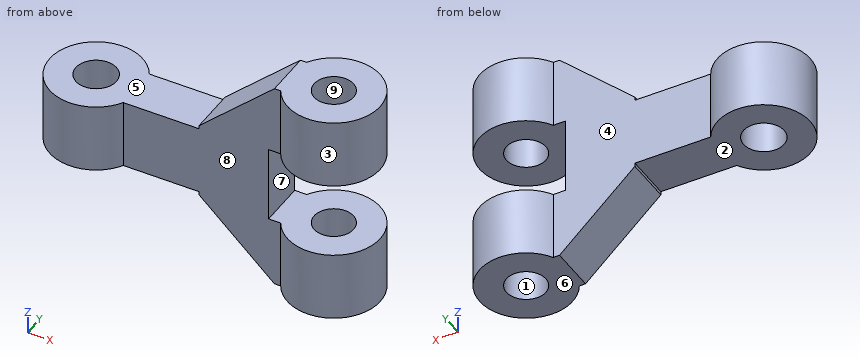
from build123d import *

# Parameters (mm, degrees)
SKETCH_1_R           = 4
SKETCH_1_R_2         = 1.7
EXTRUDE_1_DEPTH      = 6
EXTRUDE_2_DEPTH      = 2
EXTRUDE_2_DEPTH_BACK = 2
SKETCH_3_R           = 1.75
EXTRUDE_3_DEPTH      = 3
EXTRUDE_3_DEPTH_BACK = 3


with BuildPart() as part:
    # Sketch 1 → Extrude 1 (new body)
    with BuildSketch(Plane.XY):
        Circle(SKETCH_1_R)
        Circle(SKETCH_1_R_2, mode=Mode.SUBTRACT)
    extrude_1 = extrude(amount=EXTRUDE_1_DEPTH)

    # Sketch 2 → Extrude 2 (add, two sides)
    with BuildSketch(Plane(origin=(0, 0, 0), x_dir=(1, 0, 0), z_dir=(0, 1, 0))) as extrude_2_sk:
        Polygon((-4, 0), (-10.5, -6), (-10.5, -12.6), (-4, -18.6), (-3, -18.6), (-3, -12.6), (-4, -12.6), (-4.5, -12.6), (-4.5, -6), (-4, -6), (-3, -6), (-3, 0), align=None)
    extrude(amount=EXTRUDE_2_DEPTH)
    extrude(extrude_2_sk.sketch, amount=-EXTRUDE_2_DEPTH_BACK)

    # Mirror 1: Extrude 1 across plane
    add(extrude_1.mirror(Plane(origin=(0, 0, 9.3), x_dir=(1, 0, 0), z_dir=(0, 0, -1))))

    # Sketch 3 → Extrude 3 (add, two sides)
    with BuildSketch(Plane(origin=(0, 0, 9.3), x_dir=(-1, 0, 0), z_dir=(0, 0, -1))) as extrude_3_sk:
        with BuildLine():
            Line((10.5, 2), (17.035898385, 2))
            ThreePointArc((17.035898385, 2), (24.5, 0), (17.035898385, -2))
            Line((17.035898385, -2), (10.5, -2))
            Line((10.5, -2), (10.5, 2))
        make_face()
        with Locations((20.5, 0)):
            Circle(SKETCH_3_R, mode=Mode.SUBTRACT)
    extrude(amount=EXTRUDE_3_DEPTH)
    extrude(extrude_3_sk.sketch, amount=-EXTRUDE_3_DEPTH_BACK)


solid = part.part
Input: part model. Units: mm. Frame: model coordinates. Face numbers are marked on the shaded views. A direction names the side the tool comes from. Round coordinates to 2 decimals unless told otherwise and drop trailing zeros. Order: outer loops, then holes, each group sorted by start corner. A loop starts at its lowest first (then second) coordinate and runs counter-clockwise, first axis right, second up. Notation, with made-up numbers: (32, 16) - (70, 16) arc R26 cw to (70, 55) - close; hole circle Ø4 at (87.5, 74). An arc over 180 degrees is marked (long way). Answer as a JSON object with one key per item and string values. Group by question number.
(1) Material intervals for probe 1 along Z at (x, y) = (-3.25, 0.25); probe 2 along Y at (x, z) = (0, 15.1); probe 3 along X at (y, z) = (0.5, 11), sorted ascending. Write a range as from..to.
(2) Cut plane C-C (x = 0). Return loops of the section in (y, z), then the cut area to 3 significant figures.
(3) Reachability of the marked faces 5, 6, 7, 8 and 9 from +Z, -Z, +X, -X, +Y, -Y: full face, straight path, thin tool, end or side. Return the list, or none.
(4) Cut plane D-D (z = 11). Return loops of the section in (x, y).
(5) Cut plane B-B (y = 0). Return loops of the section in (x, z).
(6) Cut plane A-A (x = -20.5). Return loops of the section in (y, z), then the cut area to 3 significant figures.
(7) Draft query along Y for the marked faces 1, 2, 3 and 4. Return one class per face: released by +Y, released by -Y, zero draft, split by the parting line, or undercut.
(8) Pin query (flat end, axial travel): P1, Ø2, axis at y = -0.5, z = 10.5, coming from the +X side; P2, Ø4, axis at x = -13, z = 9.5, coming from the +Y side; P3, Ø4, axis at x = -10.5, z = 15, coming from the -Y side. Return the tip coordinate at first contact, or that it passes through.
Here are the results:
{
 "1": {"probe 1": "z = 0..6, 12.6..18.6", "probe 2": "y = -4..-1.7, 1.7..4", "probe 3": "x = -24.47..-22.18, -18.82..-4.5"},
 "2": {"outline": "(-4, 0) - (-1.7, 0) - (-1.7, 6) - (-4, 6) - close; (-4, 12.6) - (-1.7, 12.6) - (-1.7, 18.6) - (-4, 18.6) - close; (1.7, 0) - (4, 0) - (4, 6) - (1.7, 6) - close; (1.7, 12.6) - (4, 12.6) - (4, 18.6) - (1.7, 18.6) - close", "area": "55.2 mm^2"},
 "3": {"face 5": "+Z, -X, +Y, -Y", "face 6": "-Z, +X, -X, +Y, -Y", "face 7": "+X, +Y, -Y", "face 8": "+Z, -Z, -Y", "face 9": "+Z, -Z"},
 "4": {"outline": "(-17.04, -2) - (-4.5, -2) - (-4.5, 2) - (-17.04, 2) arc R4 ccw (long way) to start; hole circle Ø3.5 at (-20.5, 0)"},
 "5": {"outline": "(-24.5, 6.3) - (-22.25, 6.3) - (-22.25, 12.3) - (-24.5, 12.3) - close; (-18.75, 6.3) - (-10.5, 6.3) - (-10.5, 6) - (-4, 0) - (-1.7, 0) - (-1.7, 6) - (-4.5, 6) - (-4.5, 12.6) - (-1.7, 12.6) - (-1.7, 18.6) - (-4, 18.6) - (-10.5, 12.6) - (-10.5, 12.3) - (-18.75, 12.3) - close; (1.7, 0) - (4, 0) - (4, 6) - (1.7, 6) - close; (1.7, 12.6) - (4, 12.6) - (4, 18.6) - (1.7, 18.6) - close"},
 "6": {"outline": "(-4, 6.3) - (-1.75, 6.3) - (-1.75, 12.3) - (-4, 12.3) - close; (1.75, 6.3) - (4, 6.3) - (4, 12.3) - (1.75, 12.3) - close", "area": "27.0 mm^2"},
 "7": {"face 1": "undercut", "face 2": "zero draft", "face 3": "split by the parting line", "face 4": "released by +Y"},
 "8": {"P1": "stops at x = -4.5", "P2": "stops at y = 2", "P3": "stops at y = -2"}
}
